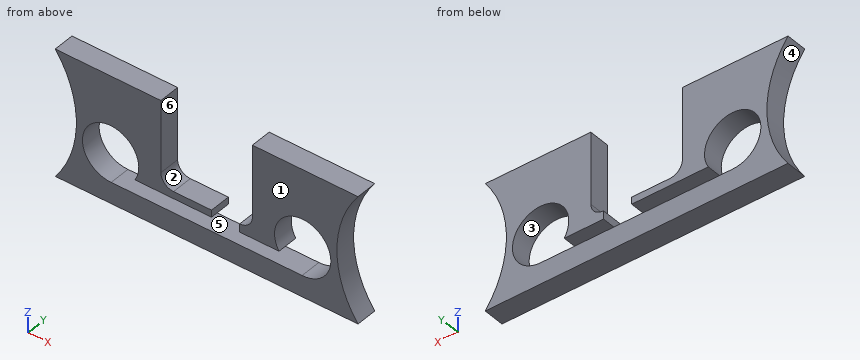
```python
from build123d import *

# Parameters (mm, degrees)
F0_W     = 273.05
F0_H     = 114.3
F1_DEPTH = 19.05
F3_DEPTH = 25.4
F4_R     = 25.4
F5_DEPTH = 25.4
F7_DEPTH = 25.4


with BuildPart() as f1:
    # F0 (on Front) → F1 (new body)
    with BuildSketch(Plane.XZ):
        with Locations((136.525, 57.15)):
            Rectangle(F0_W, F0_H)
    extrude(amount=F1_DEPTH)

    # F2 (on face) → F3 (cut)
    with BuildSketch(Plane.XZ.offset(19.05)):
        with BuildLine():
            Line((0, 114.3), (0, 0))
            ThreePointArc((0, 0), (19.05, 57.15), (0, 114.3))
        make_face()
        with BuildLine():
            ThreePointArc((273.05, 114.3), (254, 57.15), (273.05, 0))
            Line((273.05, 0), (273.05, 114.3))
        make_face()
    extrude(amount=-F3_DEPTH, mode=Mode.SUBTRACT)

    # F4 (on face) → F5 (cut)
    with BuildSketch(Plane.XZ.offset(19.05)):
        with BuildLine():
            Line((177.8, 114.3), (95.25, 114.3))
            Line((95.25, 114.3), (95.25, 49.53))
            ThreePointArc((95.25, 49.53), (106.68, 60.96), (118.11, 49.53))
            ThreePointArc((118.11, 49.53), (114.762230509, 41.447769491), (106.68, 38.1))
            Line((106.68, 38.1), (166.37, 38.1))
            ThreePointArc((166.37, 38.1), (158.287769491, 57.612230509), (177.8, 49.53))
            Line((177.8, 49.53), (177.8, 114.3))
        make_face()
        with Locations((49.9111476386, 44.45)):
            Circle(F4_R)
        with Locations((223.1418776763, 44.45)):
            Circle(F4_R)
        with BuildLine():
            ThreePointArc((166.37, 38.1), (174.452230509, 41.447769491), (177.8, 49.53))
            ThreePointArc((177.8, 49.53), (158.287769491, 57.612230509), (166.37, 38.1))
        make_face()
        with BuildLine():
            ThreePointArc((118.11, 49.53), (106.68, 60.96), (95.25, 49.53))
            ThreePointArc((95.25, 49.53), (98.597769491, 41.447769491), (106.68, 38.1))
            ThreePointArc((106.68, 38.1), (114.762230509, 41.447769491), (118.11, 49.53))
        make_face()
    extrude(amount=-F5_DEPTH, mode=Mode.SUBTRACT)

    # F6 (on face) → F7 (cut)
    with BuildSketch(Plane.XZ.offset(19.05)):
        with BuildLine():
            Line((166.37, 30.7134911418), (166.37, 38.1))
            Line((166.37, 38.1), (140.97, 38.1))
            Line((140.97, 38.1), (140.97, 31.755262097))
            Line((140.97, 31.755262097), (71.9112301288, 31.755262097))
            ThreePointArc((71.9112301288, 31.755262097), (62.8369832957, 22.5848960084), (50.4281455484, 19.055262097))
            Line((50.4281455484, 19.055262097), (222.6248797665, 19.055262097))
            ThreePointArc((222.6248797665, 19.055262097), (210.7448885281, 22.2807722269), (201.7767583369, 30.7134911418))
            Line((201.7767583369, 30.7134911418), (166.37, 30.7134911418))
        make_face()
    extrude(amount=-F7_DEPTH, mode=Mode.SUBTRACT)


solid = f1.part
```
The model under review builds one solid part; all positions refer to its coordinate system, in mm. Face numbers are marked on the shaded views. A direction names the side the tool comes from. Round coordinates to 2 decimals unless told otherwise and drop trailing zeros. Order: outer loops, then holes, each group sorted by start corner. A loop starts at its lowest first (then second) coordinate and runs counter-clockwise, first axis right, second up. Notation, with made-up numbers: (52.5, 63) -> (58.5, 63) arc R17 cw to (58.5, 72) -> close; hole circle Ø9 at (17, -28.5). An arc over 180 degrees is marked (long way). One line per item, written item: value. Start each with the question number.
Q1. Take a section at D-D (y = -15.5). Write out the cut boundary in (x, z).
Q2. Take a section at C-C (z = 22). Write out the cut boundary in (x, y).
Q3. Mouldability with a two-part tool opening along Z and no side actions: class the marked faces 1, 2 and 3 as released by +Z, released by -Z, zero draft, split by the parting line, or undercut.
Q4. Take a section at B-B (x = 240). Write out the cut boundary in (y, z), and give its area (3 significant figures).
Q5. Take a section at A-A (z = 44). Write out the cut boundary in (x, y).
Q6. Clearance check with flat-ended pins moving along their axes: pin 1 Ø4 at (y, z) = (-13, 57.5) entering from -X; pin 2 Ø3.5 at (y, z) = (-5.5, 33) entering from -X; pin 3 Ø5 at (y, z) = (-7, 23.5) entering from -X; pin 4 Ø9.5 at (x, y) = (178, -10) entering from -Z. State where each tip first meets the part, or that it passes through.
Q7. Wall thickness on line 1 (Z direction, x = 131.5, y = -5); line 2 (X direction, y = -14.5, z = 55.5); line 3 (X direction, y = -12.25, z = 44.45): over which ranges is each line inside the solid? List them lowest first.
Q8. Machinability: for the marked faces 4, 5 and 6, which of the approach directions +Z, -Z, +X, -X, +Y, -Y give a long, thin tool a straight path to every point of the face, cutting with its end or side? Answer none if there is none.
Reported:
1. outline: (0, 0) -> (273.05, 0) arc R95.25 cw to (273.05, 114.3) -> (177.8, 114.3) -> (177.8, 49.53) arc R11.43 cw to (166.37, 38.1) -> (166.37, 30.71) -> (201.78, 30.71) arc R25.4 cw (long way) to (222.62, 19.06) -> (50.43, 19.06) arc R25.4 cw (long way) to (71.91, 31.76) -> (140.97, 31.76) -> (140.97, 38.1) -> (106.68, 38.1) arc R11.43 cw to (95.25, 49.53) -> (95.25, 114.3) -> (0, 114.3) arc R95.25 cw to start
2. outline: (12.33, -19.05) -> (38.03, -19.05) -> (38.03, 0) -> (12.33, 0) -> close; (235.02, -19.05) -> (260.72, -19.05) -> (260.72, 0) -> (235.02, 0) -> close
3. face 1: zero draft
3. face 2: released by +Z
3. face 3: undercut
4. outline: (-19.05, 0) -> (0, 0) -> (0, 25.45) -> (-19.05, 25.45) -> close; (-19.05, 63.45) -> (0, 63.45) -> (0, 114.3) -> (-19.05, 114.3) -> close
4. area: 1,450 mm2
5. outline: (18.14, -19.05) -> (24.52, -19.05) -> (24.52, 0) -> (18.14, 0) -> close; (75.31, -19.05) -> (96.68, -19.05) -> (96.68, 0) -> (75.31, 0) -> close; (176.37, -19.05) -> (197.75, -19.05) -> (197.75, 0) -> (176.37, 0) -> close; (248.54, -19.05) -> (254.91, -19.05) -> (254.91, 0) -> (248.54, 0) -> close
6. pin 1: stops at x = 19.02
6. pin 2: stops at x = 15.46
6. pin 3: stops at x = 11.92
6. pin 4: stops at z = 0
7. line 1: z = 0 to 19.06, 31.76 to 38.1
7. line 2: x = 19.04 to 27.04, 72.78 to 95.25, 177.8 to 200.27, 246.01 to 254.01
7. line 3: x = 18.2 to 24.51, 75.31 to 96.44, 176.61 to 197.74, 248.54 to 254.85
8. face 4: -X, +Y, -Y
8. face 5: +Y, -Y
8. face 6: +Z, +Y, -Y
